Check sheet for the modelled part. Datum: model origin and axes. Units: mm. Round coordinates to 2 decimals unless told otherwise and drop trailing zeros. Loops run counter-clockwise (first coordinate to the right, second up) from the corner with the lowest first, then second, coordinate; pieces in that order, holes last. Notation, with made-up numbers: (19, -19.75) - (30, -19.75) arc R12 cw to (30, -13.75) - close; hole circle Ø7 at (55, 59). An arc over 180 degrees is marked (long way). Put each result on its own line as item: value.
```python
from build123d import *

# Parameters (mm, degrees)
F1_DEPTH = 12.7
F3_DEPTH = 12.701
F5_DEPTH = 25.4


with BuildPart() as f1:
    # F0 (on Top) → F1 (new body)
    with BuildSketch(Plane.XY):
        Polygon((349.925731, -349.925731), (494.869714, 0), (349.925731, 349.925731), (0, -494.869714), align=None)
    extrude(amount=F1_DEPTH)

    # F2 (on face) → F3 (cut, through all)
    with BuildSketch(Plane.XY.offset(12.7)):
        with BuildLine():
            ThreePointArc((43.288021, -466.629443), (44.712917, -465.460061), (45.248001, -463.696126))
            ThreePointArc((45.248001, -463.696126), (39.433085, -461.93219), (43.288021, -466.629443))
        make_face()
        with BuildLine():
            ThreePointArc((299.347591, -360.566096), (300.772487, -359.396714), (301.307571, -357.632779))
            ThreePointArc((301.307571, -357.632779), (295.492655, -355.868843), (299.347591, -360.566096))
        make_face()
        with BuildLine():
            ThreePointArc((360.566096, -299.347591), (360.746772, -298.751982), (360.807779, -298.132571))
            ThreePointArc((360.807779, -298.132571), (358.252191, -295.018577), (354.699461, -296.917551))
            Line((354.699461, -296.917551), (357.632779, -298.132571))
            Line((357.632779, -298.132571), (360.566096, -299.347591))
        make_face()
        with BuildLine():
            Line((357.632779, -298.132571), (354.699461, -296.917551))
            ThreePointArc((354.699461, -296.917551), (356.417759, -301.065888), (360.566096, -299.347591))
            Line((360.566096, -299.347591), (357.632779, -298.132571))
        make_face()
        with BuildLine():
            ThreePointArc((466.629443, -43.288021), (466.810119, -42.692412), (466.871126, -42.073001))
            ThreePointArc((466.871126, -42.073001), (464.315537, -38.959007), (460.762808, -40.857981))
            Line((460.762808, -40.857981), (463.696126, -42.073001))
            Line((463.696126, -42.073001), (466.629443, -43.288021))
        make_face()
        with BuildLine():
            Line((463.696126, -42.073001), (460.762808, -40.857981))
            ThreePointArc((460.762808, -40.857981), (462.481106, -45.006318), (466.629443, -43.288021))
            Line((466.629443, -43.288021), (463.696126, -42.073001))
        make_face()
        with BuildLine():
            ThreePointArc((466.629443, 43.288021), (460.582132, 41.453589), (466.871126, 42.073001))
            ThreePointArc((466.871126, 42.073001), (466.810119, 42.692412), (466.629443, 43.288021))
        make_face()
        with BuildLine():
            ThreePointArc((360.566096, 299.347591), (354.518786, 297.513159), (360.807779, 298.132571))
            ThreePointArc((360.807779, 298.132571), (360.746772, 298.751982), (360.566096, 299.347591))
        make_face()
    extrude(amount=-F3_DEPTH, mode=Mode.SUBTRACT)

    # F4 (on face) → F5 (cut)
    with BuildSketch(Plane.XY.offset(12.7)):
        Polygon((230.305284, -52.50727), (195.584189, -147.990282), (207.519565, -152.330419), (242.24066, -56.847407), align=None)
    extrude(amount=-F5_DEPTH, mode=Mode.SUBTRACT)


solid = f1.part
```
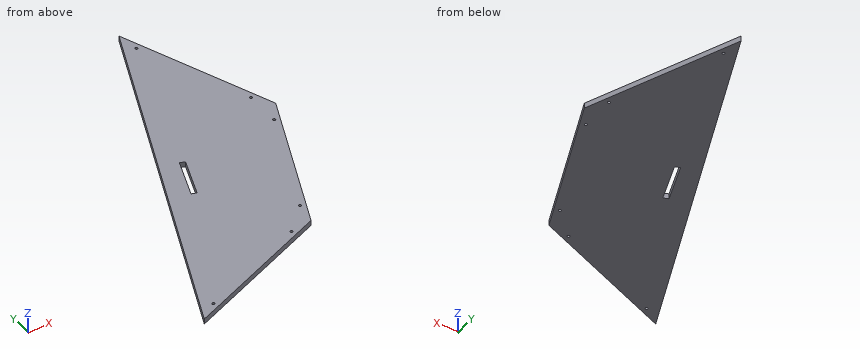
Item 1: Section check C-C on y = 23.5. Enter the section's corners in (x, z), then the cut area to 3 significant figures.
Filled sheet:
outline: (214.72, 0) - (485.14, 0) - (485.14, 12.7) - (214.72, 12.7) - close
area: 3,430 mm²
Item 2: Go/stop test with flat-tipped pins: pin 1 (1 mm diameter, centred on x = 149.5, z = 9, fed in from +Y); pin 2 (3 mm diameter, centred on x = 312, y = -8.5, fed in from -Z); pin 3 (4 mm diameter, centred on x = 463.7, y = 42.07, fed in from -Z); pin 4 (6 mm diameter, centred on x = 354.5, z = 9.5, fed in from +Y). Record where each tip stops, or that it passes through.
Filled sheet:
pin 1: y = -132.74
pin 2: z = 0
pin 3: through
pin 4: y = 346.13
Item 3: Section check B-B on x = 386.5. Enter the section's corners in (y, z).
Filled sheet:
outline: (-261.63, 0) - (261.63, 0) - (261.63, 12.7) - (-261.63, 12.7) - close
Item 4: Thickness scan on line 1 (Y direction, x = 461, z = 1.5); line 2 (X direction, y = -102, z = 8.5); line 3 (X direction, y = -100, z = 8.25). Record the ranges inside material, lowest first. Write a range as from..to.
Filled sheet:
line 1: -81.77..-43.75, -40.4..40.4, 43.75..81.77
line 2: 162.73..212.31, 225.82..452.62
line 3: 163.56..213.04, 226.55..453.45
Item 5: Section check A-A on z = 9.5. Enter the section's corners in (x, y) (3 decimals), then the cut area to 3 significant figures.
Filled sheet:
outline: (0, -494.87) - (349.926, -349.926) - (494.87, 0) - (349.926, 349.926) - close; hole circle Ø6.35 at (42.073, -463.696); hole (195.584, -147.99) - (207.52, -152.33) - (242.241, -56.847) - (230.305, -52.507) - close; hole circle Ø6.35 at (298.133, -357.633); hole (360.566, -299.348) arc R3.175 ccw to (360.808, -298.133) arc R3.175 ccw (long way) to start; hole (360.566, 299.348) arc R3.175 ccw (long way) to (360.808, 298.133) arc R3.175 ccw to start; hole (466.629, -43.288) arc R3.175 ccw to (466.871, -42.073) arc R3.175 ccw (long way) to start; hole (466.629, 43.288) arc R3.175 ccw (long way) to (466.871, 42.073) arc R3.175 ccw to start
area: 172,000 mm²
